Solid Edge part; units mm, degrees
sketch "Sketch1" plane through (0, 0, 0) normal (0, -1, 0) x (1, 0, 0)
  line L0 (-2.5, -0.795) -> (2.5, -0.795)
  line L1 (2.5, -0.795) -> (2.5, 0.795)
  line L2 (2.5, 0.795) -> (-2.5, 0.795)
  line L3 (-2.5, 0.795) -> (-2.5, -0.795)
extrude "Protrusion1" add sketch "Sketch1" along normal mid plane 34
fillet "Round_2" radius 2.5 4 edges at (-2.5, -17, 0) (2.5, -17, 0) (2.5, 17, 0) (-2.5, 17, 0)
hole "Hole_1" at (0, 0, 0.795) direction (0, 0, -1) diameter 3.6 end through all
Model file for the job. Use its own axes, mm. Coordinates: 2 decimals unless noted, no trailing zeros. Loops run counter-clockwise (first coordinate to the right, second up) from the corner with the lowest first, then second, coordinate; pieces in that order, holes last. Notation, with made-up numbers: M 80,57 L 91,57 A14 cw 91,80 Z; hole C 24.25,60 d6. An arc over 180 degrees is marked long. Use CSV: the item, a comma, the result in double quotes. Start each with the question number.
1. Probe probe 1 along X at (y, z) = (0, 0.25); probe 2 along Y at (x, z) = (0, 0.1); probe 3 along Y at (x, z) = (-1.1, 0.75). List the from-to ranges inside material, lowest first. Write a range as [from, to].
2. Band-saw the part on B-B, the plane x = -0.5. List the corners of the cut face in (y, z) (3 decimals), then the cut area to 3 significant figures.
3. Two-plate mould, pull along X, no slides. Class faces 1 (the flat face through (-2, 0, 0.795)), 2 (the cylindrical face through (0.541, -1.717, 0.011)), 3 (the cylindrical face through (-2, -16, 0)): pulls with the +X half, pulls with the -X half, needs draft (parallel to the pull), parting line crosses it, or undercut.
4. Band-saw the part on A-A, the plane y = 0. List the corners of the cut face in (x, z) (3 decimals), then the cut area to 3 significant figures.
Entries:
1,probe 1,"x = [-2.5, -1.8], [1.8, 2.5]"
1,probe 2,"y = [-17, -1.8], [1.8, 17]"
1,probe 3,"y = [-16.75, -1.42], [1.42, 16.75]"
2,outline,"M -16.95,-0.795 L -1.729,-0.795 L -1.729,0.795 L -16.95,0.795 Z; M 1.729,-0.795 L 16.95,-0.795 L 16.95,0.795 L 1.729,0.795 Z"
2,area,"48.4 mm2"
3,face 1,"needs draft"
3,face 2,"undercut"
3,face 3,"pulls with the -X half"
4,outline,"M -2.5,-0.795 L -1.8,-0.795 L -1.8,0.795 L -2.5,0.795 Z; M 1.8,-0.795 L 2.5,-0.795 L 2.5,0.795 L 1.8,0.795 Z"
4,area,"2.23 mm2"
